Design review of the part shown in the three views and the two pictorial views. Dimensions are in mm from the part's minimum x, y and z. A direction names the side the tool comes from. Coordinates: 2 decimals unless noted, no trailing zeros. Write each loop counter-clockwise with the first axis right and the second up, starting at its lowest first coordinate (ties: lowest second). Pieces come first, ordered by that corner, then holes. Notation, with made-up numbers: (12, 17) - (63, 17) arc R15 cw to (63, 24) - close; hole circle Ø3 at (6.25, 10). An arc over 180 degrees is marked (long way). Write each question's results on one line, items separated by ' | '.
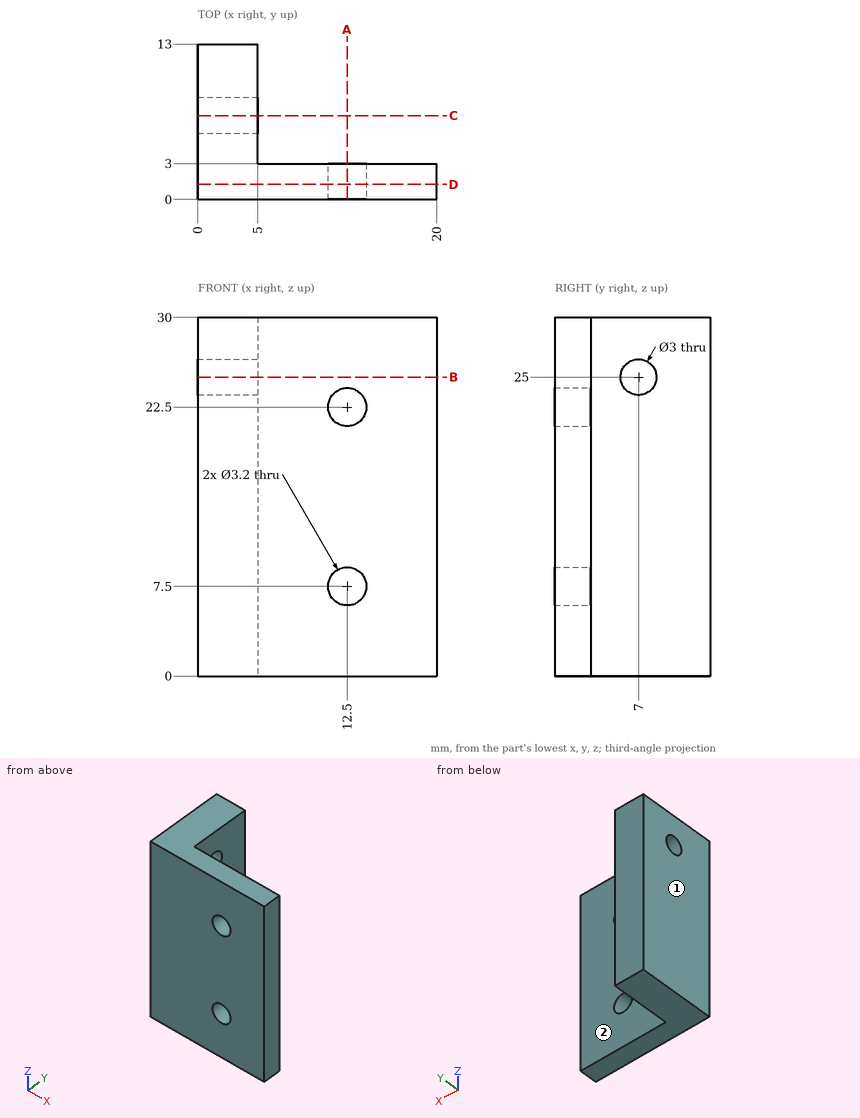
Q1. Wall thickness on line 1 along Z through (x, y) = (12.5, 1.9); line 2 along X through (y, z) = (2.1, 7.5); line 3 along Y through (x, z) = (9.25, 23.5): over which ranges is each line inside the solid? List them lowest first. Write a range as from..to.
Results found:
line 1: 0..5.9, 9.1..20.9, 24.1..30 | line 2: 0..10.9, 14.1..20 | line 3: 0..3
Q2. Take a section at D-D on y = 1.25. State the section outline as (x, z) points, plus the area to 3 significant figures.
Results found:
outline: (0, 0) - (20, 0) - (20, 30) - (0, 30) - close; hole circle Ø3.2 at (12.5, 7.5); hole circle Ø3.2 at (12.5, 22.5) | area: 584 mm2
Q3. For pin 1 (5 mm diameter, centred on y = 8, z = 16.5, fed in from +X); pin 2 (5 mm diameter, centred on x = 15, z = 14.5, fed in from +Y), all flat-tipped, find the tip position at first contact; note any pin that passes through.
Results found:
pin 1: x = 5 | pin 2: y = 3
Q4. For the marked faces 1 and 2, list the 3-axis set-ups (+Z, -Z, +X, -X, +Y, -Y) from which the entire face can be reached by the end or side of a thin tool; tool diameter is ignored.
Results found:
face 1: +Z, -Z, -X, +Y, -Y | face 2: +Z, -Z, +X, +Y
Q5. Take a section at A-A on x = 12.5. State the section outline as (y, z) points.
Results found:
outline: (0, 0) - (3, 0) - (3, 5.9) - (0, 5.9) - close; (0, 9.1) - (3, 9.1) - (3, 20.9) - (0, 20.9) - close; (0, 24.1) - (3, 24.1) - (3, 30) - (0, 30) - close
Q6. Take a section at C-C on y = 7. State the section outline as (x, z) points, plus the area to 3 significant figures.
Results found:
outline: (0, 0) - (5, 0) - (5, 23.5) - (0, 23.5) - close; (0, 26.5) - (5, 26.5) - (5, 30) - (0, 30) - close | area: 135 mm2
Q7. Take a section at B-B on z = 25. State the section outline as (x, y) points, plus the area to 3 significant figures.
Results found:
outline: (0, 0) - (20, 0) - (20, 3) - (5, 3) - (5, 5.5) - (0, 5.5) - close; (0, 8.5) - (5, 8.5) - (5, 13) - (0, 13) - close | area: 95.0 mm2
